Part model, mm, in its own coordinate system. A direction names the side the tool comes from. Round coordinates to 2 decimals unless told otherwise and drop trailing zeros. Write each loop counter-clockwise with the first axis right and the second up, starting at its lowest first coordinate (ties: lowest second). Pieces come first, ordered by that corner, then holes. Notation, with made-up numbers: M 72.25,47 L 124.25,47 A35 ccw 124.25,81 Z; hole C -18,-32 d3. An arc over 180 degrees is marked long. Use one line per item in the form item = value. Start each with the question number.
Item 1: Cut at A-A, the plane x = 42. Give the cut face in (y, z).
Item 2: Cut at D-D, the plane y = -2. State how many separate pieces and enclosed holes the cut face has, then the cut area to 3 significant figures.
Item 3: Cut at B-B, the plane x = -30. Give the cut face in (y, z), then the cut area to 3 significant figures.
Item 4: Which spindle directions (+Z, -Z, +X, -X, +Y, -Y) get a long thin tool onto all of the face, cutting with end or side? Do faces 4 (the face through (20, -2, 32)), 5 (the face through (-83, -2, -25)), 6 (the face through (-20, -2, -32)). Say none if no direction does.
Item 5: Mould opens along X. For faces 1 (the face through (-60, -2, -32)), 2 (the face through (70, -1, 35)), 3 (the face through (-75, -2, -34)) say: +X half, -X half, draft (parallel to the pull), parting line (faces both ways), or undercut.
Item 6: Probe L1, parallel to Z at x = 66, y = -2.3; L2, parallel to Z at x = -42, y = -2.3; L3, parallel to Z at x = -58, y = -1.1. List the from-to ranges inside material, lowest first.
Item 7: Cut at C-C, the plane z = 28.5. Give the cut face in (x, y), then the cut area to 3 significant figures.
Item 8: Flat gauge pins, fed straight in: pin 1 Ø0.9 at (y, z) = (-1, 33.5) entering from -X; pin 2 Ø1.5 at (x, y) = (22, -1.5) entering from -Z; pin 3 Ø0.9 at (x, y) = (83, -1) entering from -Z. Where does each tip first touch, or does it go through?
from build123d import *

# Parameters (mm, degrees)
F0_W     = 170
F0_H     = 70
F1_DEPTH = 3
F2_R     = 3
F3_DEPTH = 3.001
F4_R     = 1.5
F5_DEPTH = 3.001
F6_R     = 1.5
F7_DEPTH = 3.001
F8_W     = 3
F8_H     = 3
F8_W_2   = 7
F8_W_3   = 10
F8_H_2   = 7
F9_DEPTH = 3.001


with BuildPart() as f1:
    # F0 (on Front) → F1 (new body)
    with BuildSketch(Plane.XZ):
        Rectangle(F0_W, F0_H)
    extrude(amount=F1_DEPTH)

    # F2 (on face) → F3 (cut, through all)
    with BuildSketch(Plane.XZ.offset(3)):
        with Locations((66, -15)):
            Circle(F2_R)
        with Locations((54, -15)):
            Circle(F2_R)
        with Locations((42, -15)):
            Circle(F2_R)
        with Locations((30, -15)):
            Circle(F2_R)
        with Locations((18, -15)):
            Circle(F2_R)
        with Locations((6, -15)):
            Circle(F2_R)
        with Locations((-6, -15)):
            Circle(F2_R)
        with Locations((-18, -15)):
            Circle(F2_R)
        with Locations((-30, -15)):
            Circle(F2_R)
        with Locations((-42, -15)):
            Circle(F2_R)
        with Locations((-54, -15)):
            Circle(F2_R)
        with Locations((-66, -15)):
            Circle(F2_R)
    extrude(amount=-F3_DEPTH, mode=Mode.SUBTRACT)

    # F4 (on face) → F5 (cut, through all)
    with BuildSketch(Plane.XZ.offset(3)):
        with Locations((-66, -2)):
            Circle(F4_R)
        with Locations((-54, -2)):
            Circle(F4_R)
        with Locations((-42, -2)):
            Circle(F4_R)
        with Locations((-30, -2)):
            Circle(F4_R)
        with Locations((-18, -2)):
            Circle(F4_R)
        with Locations((-6, -2)):
            Circle(F4_R)
        with Locations((6, -2)):
            Circle(F4_R)
        with Locations((18, -2)):
            Circle(F4_R)
        with Locations((30, -2)):
            Circle(F4_R)
        with Locations((42, -2)):
            Circle(F4_R)
        with Locations((54, -2)):
            Circle(F4_R)
        with Locations((66, -2)):
            Circle(F4_R)
    extrude(amount=-F5_DEPTH, mode=Mode.SUBTRACT)

    # F6 (on face) → F7 (cut, through all)
    with BuildSketch(Plane.XZ.offset(3)):
        with Locations((54, 13.5)):
            Circle(F6_R)
        with Locations((54, 23.5)):
            Circle(F6_R)
    extrude(amount=-F7_DEPTH, mode=Mode.SUBTRACT)

    # F8 (on face) → F9 (cut, through all)
    with BuildSketch(Plane.XZ.offset(3)):
        with Locations((-83.5, -33.5)):
            Rectangle(F8_W, F8_H)
        with Locations((-78.5, -33.5)):
            Rectangle(F8_W_2, F8_H)
        Polygon((-85, -28), (-85, -32), (-82, -32), (-82, -25), (-85, -25), align=None)
        with Locations((-60, -33.5)):
            Rectangle(F8_W_3, F8_H)
        with Locations((-40, -33.5)):
            Rectangle(F8_W_3, F8_H)
        with Locations((-20, -33.5)):
            Rectangle(F8_W_3, F8_H)
        with Locations((0, -33.5)):
            Rectangle(F8_W_3, F8_H)
        with Locations((20, -33.5)):
            Rectangle(F8_W_3, F8_H)
        with Locations((40, -33.5)):
            Rectangle(F8_W_3, F8_H)
        with Locations((60, -33.5)):
            Rectangle(F8_W_3, F8_H)
        with Locations((83.5, -33.5)):
            Rectangle(F8_W, F8_H)
        Polygon((82, -32), (85, -32), (85, -28), (85, -25), (82, -25), align=None)
        with Locations((78.5, -33.5)):
            Rectangle(F8_W_2, F8_H)
        with Locations((-60, 33.5)):
            Rectangle(F8_W_3, F8_H)
        with Locations((-20, 33.5)):
            Rectangle(F8_W_3, F8_H)
        with Locations((-40, 33.5)):
            Rectangle(F8_W_3, F8_H)
        with Locations((0, 33.5)):
            Rectangle(F8_W_3, F8_H)
        with Locations((-83.5, 33.5)):
            Rectangle(F8_W, F8_H)
        with Locations((-83.5, 28.5)):
            Rectangle(F8_W, F8_H_2)
        with Locations((-78.5, 33.5)):
            Rectangle(F8_W_2, F8_H)
        with Locations((78.5, 33.5)):
            Rectangle(F8_W_2, F8_H)
        with Locations((83.5, 33.5)):
            Rectangle(F8_W, F8_H)
        with Locations((83.5, 28.5)):
            Rectangle(F8_W, F8_H_2)
        with Locations((20, 33.5)):
            Rectangle(F8_W_3, F8_H)
        with Locations((40, 33.5)):
            Rectangle(F8_W_3, F8_H)
        with Locations((60, 33.5)):
            Rectangle(F8_W_3, F8_H)
        Polygon((-82, 5), (-82, 15), (-85, 15), (-85, 12), (-85, 5), align=None)
        Polygon((-82, -15), (-82, -5), (-85, -5), (-85, -8), (-85, -15), align=None)
        Polygon((85, 12), (85, 15), (82, 15), (82, 5), (85, 5), align=None)
        Polygon((85, -8), (85, -5), (82, -5), (82, -15), (85, -15), align=None)
    extrude(amount=-F9_DEPTH, mode=Mode.SUBTRACT)


solid = f1.part
Model answer:
q1.outline = M -3,-32 L 0,-32 L 0,-18 L -3,-18 Z; M -3,-12 L 0,-12 L 0,-3.5 L -3,-3.5 Z; M -3,-0.5 L 0,-0.5 L 0,32 L -3,32 Z
q2.separate_pieces = 1
q2.enclosed_holes = 26
q2.area = 10,700 mm²
q3.outline = M -3,-35 L 0,-35 L 0,-18 L -3,-18 Z; M -3,-12 L 0,-12 L 0,-3.5 L -3,-3.5 Z; M -3,-0.5 L 0,-0.5 L 0,35 L -3,35 Z
q3.area = 183 mm²
q4.face_4 = +Z, +Y, -Y
q4.face_5 = -Z, -X, +Y, -Y
q4.face_6 = -Z, +Y, -Y
q5.face_1 = undercut
q5.face_2 = draft
q5.face_3 = -X half
q6.L1 = -35 to -18, -12 to -3.5, -0.5 to 35
q6.L2 = -32 to -18, -12 to -3.5, -0.5 to 32
q6.L3 = -32 to 32
q7.outline = M -82,-3 L 82,-3 L 82,0 L -82,0 Z
q7.area = 492 mm²
q8.pin_1 = -75
q8.pin_2 = -32
q8.pin_3 = -25
